Part print with two shaded views. Sizes in mm from the minimum x, y, z corner. Round coordinates to 2 decimals unless told otherwise and drop trailing zeros. Order: outer loops, then holes, each group sorted by start corner. A loop starts at its lowest first (then second) coordinate and runs counter-clockwise, first axis right, second up. Notation, with made-up numbers: (48, -35) -> (88, -35) arc R25 cw to (88, -12) -> close; hole circle Ø10 at (15, 28). An arc over 180 degrees is marked (long way). Use a Markdown table: item, result. Add a question column.
Item 1: Slice it at D-D, the plane y = 40. Give the cut face in (x, z), plus the area to 3 significant figures.
Item 2: Slice it at B-B, the plane x = 6.25. Give the cut face in (y, z), plus the area to 4 significant figures.
Item 3: Pin check, flat tips, straight feed: pin 1 (1.5 mm diameter, centred on x = 24.5, z = 2, fed in from +Y); pin 2 (1.5 mm diameter, centred on y = 7, z = 1, fed in from -X); pin 3 (0.9 mm diameter, centred on y = 41, z = 2, fed in from +X). Stop position of each tip, or through.
Item 4: Probe L1, parallel to Y at x = 28, z = 1.15; L2, parallel to Y at x = 6.25, z = 1.7; L3, parallel to X at y = 62.5, z = 1.7. List the from-to ranges inside material, lowest first.
Item 5: Slice it at C-C, the plane z = 2.2. Give the cut face in (x, y).
Item 6: Slice it at A-A, the plane y = 12. Give the cut face in (x, z).
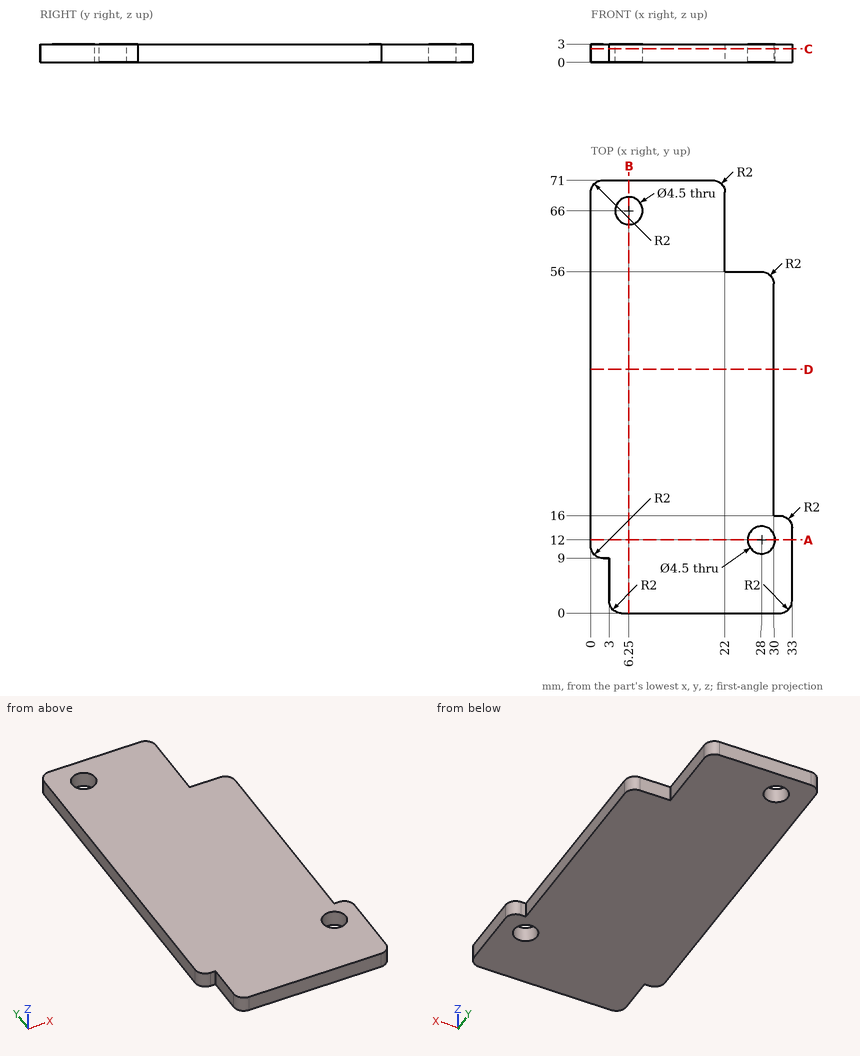
Check sheet entries:
| question | item | result |
|---|---|---|
| 1 | outline | (0, 0) -> (30, 0) -> (30, 3) -> (0, 3) -> close |
| 1 | area | 90.0 mm2 |
| 2 | outline | (0, 0) -> (63.75, 0) -> (63.75, 3) -> (0, 3) -> close; (68.25, 0) -> (71, 0) -> (71, 3) -> (68.25, 3) -> close |
| 2 | area | 199.5 mm2 |
| 3 | pin 1 | y = 56 |
| 3 | pin 2 | x = 3 |
| 3 | pin 3 | x = 30 |
| 4 | L1 | 0 to 9.75, 14.25 to 56 |
| 4 | L2 | 0 to 63.75, 68.25 to 71 |
| 4 | L3 | 0 to 22 |
| 5 | outline | (0, 11) arc R2 ccw to (2, 9) -> (3, 9) -> (3, 2) arc R2 ccw to (5, 0) -> (31, 0) arc R2 ccw to (33, 2) -> (33, 14) arc R2 ccw to (31, 16) -> (30, 16) -> (30, 54) arc R2 ccw to (28, 56) -> (22, 56) -> (22, 69) arc R2 ccw to (20, 71) -> (2, 71) arc R2 ccw to (0, 69) -> close; hole circle Ø4.5 at (6.25, 66); hole circle Ø4.5 at (28, 12) |
| 6 | outline | (0, 0) -> (25.75, 0) -> (25.75, 3) -> (0, 3) -> close; (30.25, 0) -> (33, 0) -> (33, 3) -> (30.25, 3) -> close |
